Verification items for the finished model (mm, model axes). A direction names the side the tool comes from. Coordinates: 2 decimals unless noted, no trailing zeros. Order: outer loops, then holes, each group sorted by start corner. A loop starts at its lowest first (then second) coordinate and runs counter-clockwise, first axis right, second up. Notation, with made-up numbers: (-21, 69) - (-4, 69) arc R14 cw to (-4, 84) - close; hole circle Ø1 at (37, -31). An arc over 180 degrees is marked (long way). Answer as CSV lines item,"result". Start each with the question number.
1. Mould release check, pull along Y, two halves, no side actions. Record for faces 5 (the cylindrical face through (0.04, -7.62, 0.06)), 6 (the flat face through (9.525, -6, 0)), 7 (the cylindrical face through (-6.31, -10.79, 4.54)), 8 (the flat face through (0, 12.7, 0)): pulls with the +Y half, pulls with the -Y half, needs draft (parallel to the pull), parting line crosses it, or undercut.
2. Section check C-C (z = -4.5). Record the cut outline in (x, y) (3 decimals), and give its area (3 significant figures).
3. Go/stop test with flat-tipped pins: pin 1 (4 mm diameter, centred on x = 2, y = -6.5, fed in from +Z); pin 2 (3 mm diameter, centred on x = 5.5, y = 6, fed in from +Z); pin 3 (14 mm diameter, centred on y = -9, z = 2.5, fed in from +X) (3 decimals). Record where each tip stops, or that it passes through.
4. Set-up check for faces 1 (the flat face through (-6, -3, 6.35)), 2 (the flat face through (-9.525, -6, 0)), 3 (the flat face through (6, -3, -6.35)), 4 (the cylindrical face through (-3.441, 6.261, -15.497)): record each of +Z, -Z, +X, -X, +Y, -Y from which the full face is reachable in a straight line by a thin tool's end or side.
5. Material ranges on L1, parallel to X at y = -7.5, z = 3 (3 decimals); L2, parallel to Y at x = 10, z = -4; L3, parallel to Z at x = -4.5, y = -6.25, recorded low to high. Write a range as [from, to].
6. Section check B-B (y = -2). Record the cut outline in (x, z) (3 decimals).
7. Section check A-A (x = 0). Record the cut outline in (y, z) (3 decimals).
from build123d import *

# Parameters (mm, degrees)
F0_R     = 15.875
F1_DEPTH = 12.7
F2_W     = 6.35
F2_H     = 12.7
F3_DEPTH = 12.7
F4_R     = 6.34999
F5_R     = 1.27
F6_DEPTH = 19.05


# Not quite as in the source:
# - a fillet or chamfer is up to 0.001 mm smaller than in the source, because OpenCascade refuses the exact size


with BuildPart() as f1:
    # F0 (on Front) → F1 (new body)
    with BuildSketch(Plane.XZ):
        Circle(F0_R)
    extrude(amount=-F1_DEPTH)

    # F2 (on face) → F3 (join)
    with BuildSketch(Plane.XZ):
        with Locations((-6.35, 0)):
            Rectangle(F2_W, F2_H)
        with Locations((6.35, 0)):
            Rectangle(F2_W, F2_H)
    extrude(amount=F3_DEPTH)

    # F4 (radius 6.35 in the source; OpenCascade refuses exactly that, so slightly less here)
    f4_edges = [f1.edges().sort_by_distance(p)[0] for p in [
        (-6.35, -12.7, 6.35),
        (6.35, -12.7, 6.35),
        (-6.35, -12.7, -6.35),
        (6.35, -12.7, -6.35),
    ]]
    fillet(f4_edges, radius=F4_R)

    # F5 (on face) → F6 (join)
    with BuildSketch(Plane.YZ.offset(9.525)):
        with Locations((-6.35, 0)):
            Circle(F5_R)
    extrude(amount=-F6_DEPTH)


solid = f1.part
Evaluation:
1,face 5,"undercut"
1,face 6,"needs draft"
1,face 7,"pulls with the -Y half"
1,face 8,"pulls with the +Y half"
2,outline,"(-15.224, 0) - (-9.525, 0) - (-9.525, -10.83) - (-3.175, -10.83) - (-3.175, 0) - (3.175, 0) - (3.175, -10.83) - (9.525, -10.83) - (9.525, 0) - (15.224, 0) - (15.224, 12.7) - (-15.224, 12.7) - close"
2,area,"524 mm²"
3,pin 1,"stops at z = 6.35"
3,pin 2,"stops at z = 15.36"
3,pin 3,"stops at x = 9.525"
4,face 1,"+Z, +X, -X, -Y"
4,face 2,"+Z, -Z, -X, -Y"
4,face 3,"-Z, +X, -X, -Y"
4,face 4,"+Y, -Y"
5,L1,"x = [-9.525, -3.175], [3.175, 9.525]"
5,L2,"y = [0, 12.7]"
5,L3,"z = [-6.35, 6.35]"
6,outline,"(-9.525, -6.35) - (-3.175, -6.35) - (-3.175, 6.35) - (-9.525, 6.35) - close; (3.175, -6.35) - (9.525, -6.35) - (9.525, 6.35) - (3.175, 6.35) - close"
7,outline,"circle Ø2.54 at (-6.35, 0); (0, -15.875) - (12.7, -15.875) - (12.7, 15.875) - (0, 15.875) - close"
